Verification items for this drawing (mm, ordinates from the low corner). Round coordinates to 2 decimals unless told otherwise and drop trailing zeros. Loops run counter-clockwise (first coordinate to the right, second up) from the corner with the lowest first, then second, coordinate; pieces in that order, holes last. Notation, with made-up numbers: (-12, -29) - (10, -29) arc R8 ccw to (10, -23) - close; hole circle Ø5 at (-39.5, -10). An arc over 180 degrees is marked (long way). Put each result on its own line as item: value.
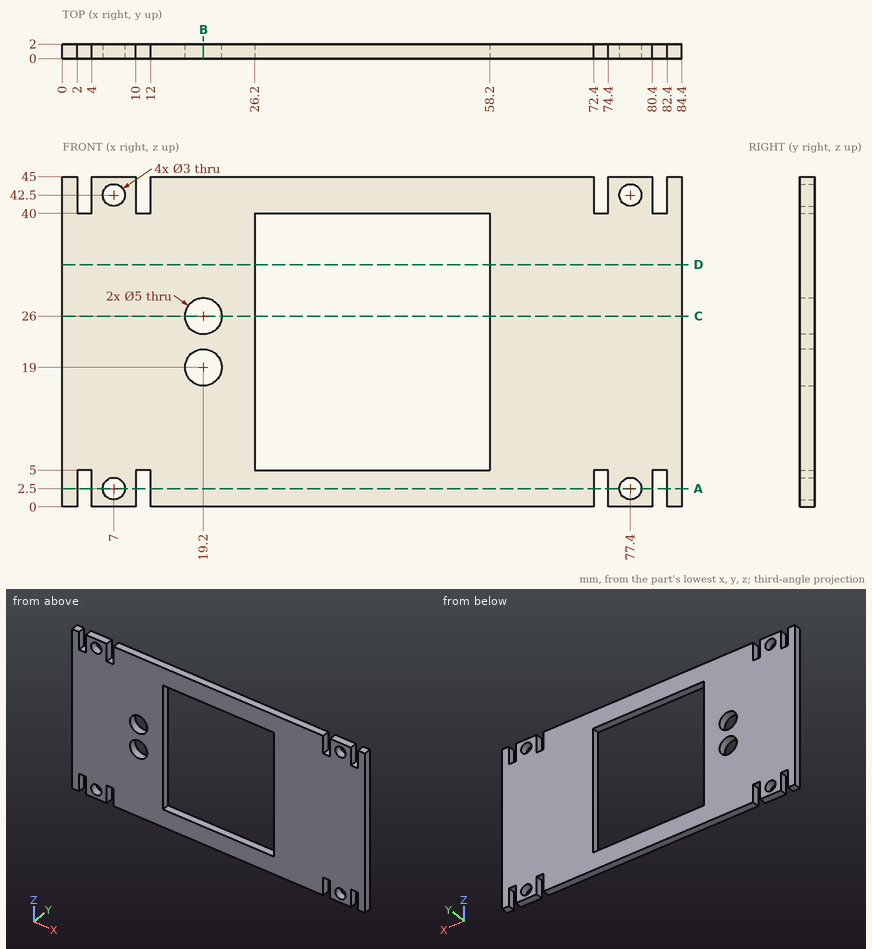
Item 1: Section check B-B on x = 19.2. Enter the section's corners in (y, z).
Filled sheet:
outline: (0, 0) - (2, 0) - (2, 16.5) - (0, 16.5) - close; (0, 21.5) - (2, 21.5) - (2, 23.5) - (0, 23.5) - close; (0, 28.5) - (2, 28.5) - (2, 45) - (0, 45) - close
Item 2: Go/stop test with a flat-tipped pin: pin 1 (0.6 mm diameter, centred on x = 81.5, y = 0.5, fed in from +Z). Record where the tip stops, or that it passes through.
Filled sheet:
pin 1: z = 40
Item 3: Section check A-A on z = 2.5. Enter the section's corners in (x, y), then the cut area to 3 significant figures.
Filled sheet:
outline: (0, 0) - (2, 0) - (2, 2) - (0, 2) - close; (4, 0) - (5.5, 0) - (5.5, 2) - (4, 2) - close; (8.5, 0) - (10, 0) - (10, 2) - (8.5, 2) - close; (12, 0) - (72.4, 0) - (72.4, 2) - (12, 2) - close; (74.4, 0) - (75.9, 0) - (75.9, 2) - (74.4, 2) - close; (78.9, 0) - (80.4, 0) - (80.4, 2) - (78.9, 2) - close; (82.4, 0) - (84.4, 0) - (84.4, 2) - (82.4, 2) - close
area: 141 mm²
Item 4: Thickness scan on line 1 (X direction, y = 0.95, z = 26); line 2 (X direction, y = 0.5, z = 36); line 3 (Z direction, x = 57.5, y = 1). Record the ranges inside material, lowest first. Write a range as from..to.
Filled sheet:
line 1: 0..16.7, 21.7..26.2, 58.2..84.4
line 2: 0..26.2, 58.2..84.4
line 3: 0..5, 40..45
Item 5: Section check D-D on z = 33. Enter the section's corners in (x, y).
Filled sheet:
outline: (0, 0) - (26.2, 0) - (26.2, 2) - (0, 2) - close; (58.2, 0) - (84.4, 0) - (84.4, 2) - (58.2, 2) - close
Item 6: Section check C-C on z = 26. Enter the section's corners in (x, y), then the cut area to 3 significant figures.
Filled sheet:
outline: (0, 0) - (16.7, 0) - (16.7, 2) - (0, 2) - close; (21.7, 0) - (26.2, 0) - (26.2, 2) - (21.7, 2) - close; (58.2, 0) - (84.4, 0) - (84.4, 2) - (58.2, 2) - close
area: 94.8 mm²
